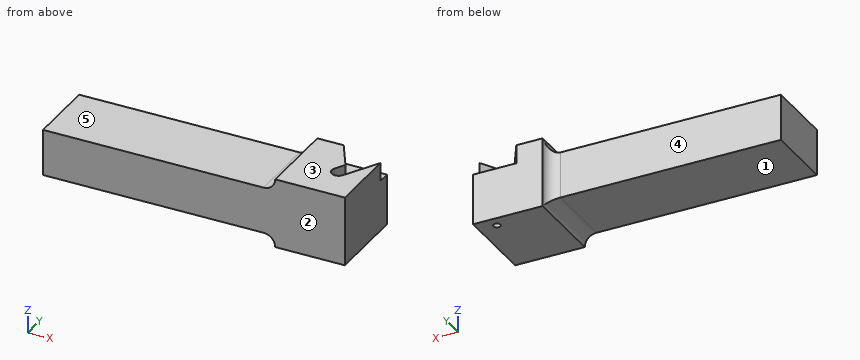
```python
from build123d import *

# Parameters (mm, degrees)
SKETCH_1_W          = 100
SKETCH_1_H          = 30
EXTRUDE_1_DEPTH     = 20
SKETCH_2_W          = 30
SKETCH_2_H          = 35
EXTRUDE_2_DEPTH     = 30
FILLET_1_R          = 5
CUT_EXTRUDE_1_DEPTH = 8
SKETCH_4_R          = 1.5
CUT_EXTRUDE_2_DEPTH = 91.049986119


with BuildPart() as part:
    # 草图1 → 凸台-拉伸1 (new body)
    with BuildSketch(Plane.XY):
        with Locations((5, 0)):
            Rectangle(SKETCH_1_W, SKETCH_1_H)
    extrude(amount=EXTRUDE_1_DEPTH)

    # 草图2 → 凸台-拉伸2 (add)
    with BuildSketch(Plane(origin=(55, 0, 0), x_dir=(0, 0, -1), z_dir=(1, 0, 0))):
        with Locations((-10, 2.5)):
            Rectangle(SKETCH_2_W, SKETCH_2_H)
    extrude(amount=EXTRUDE_2_DEPTH)

    # 圆角1
    fillet_1_edges = [part.edges().sort_by_distance(p)[0] for p in [
        (55, 0, 0),
        (55, 15, 10),
        (55, 0, 20),
    ]]
    fillet(fillet_1_edges, radius=FILLET_1_R - 0.0001)  # a hair under: the kernel refuses the full size

    # 草图3 → 切除-拉伸1 (cut)
    with BuildSketch(Plane.XY.offset(25)):
        with BuildLine():
            Line((73.842770799, 7.009618943), (66.342770799, 20))
            Line((66.342770799, 20), (85, 20))
            Line((85, 20), (85, 14.424396121))
            Line((85, 14.424396121), (78.356092757, 2.916811216))
            Line((78.356092757, 2.916811216), (76.5, -0.298035743))
            ThreePointArc((76.5, -0.298035743), (72.432621566, -1.38788651), (71.342770799, 2.679491924))
            Line((71.342770799, 2.679491924), (73.842770799, 7.009618943))
        make_face()
    extrude(amount=-CUT_EXTRUDE_1_DEPTH, mode=Mode.SUBTRACT)

    # 草图4 → 切除-拉伸2 (cut, through all)
    with BuildSketch(Plane.XY.offset(17)):
        with Locations((77.2809236, 15.014563609)):
            Circle(SKETCH_4_R)
    extrude(amount=-CUT_EXTRUDE_2_DEPTH, mode=Mode.SUBTRACT)


solid = part.part
```
Work out the finished part from the listing and answer in its coordinate system (mm). Face numbers are marked on the shaded views. A direction names the side the tool comes from. Give positions to 0.01 mm unless a question says otherwise; leave off trailing zeros. Write each loop counter-clockwise with the first axis right and the second up, starting at its lowest first coordinate (ties: lowest second). Pieces come first, ordered by that corner, then holes.
(1) The part is cut by section D-D on x = -35. Write down the section's boundary in (y, z).
Final values:
outline: (-15, 0) - (15, 0) - (15, 20) - (-15, 20) - close
(2) Straight lines are drawn through the part: line 1 (Z direction, x = -25.5, y = 1); line 2 (Y direction, x = 44.5, z = 1); line 3 (Y direction, x = 76.5, z = 13). For each, find the intervals that lie inside material, in ascending order.
Final values:
line 1: z = 0 to 20
line 2: y = -15 to 15
line 3: y = -15 to 13.73, 16.3 to 20
(3) Flat-ended cylindrical pins translate along their axes: pin 1 Ø8 at (x, y) = (18, -8) entering from -Z; pin 2 Ø16 at (x, z) = (25.5, 12.5) entering from +Y; pin 3 Ø9 at (x, y) = (18.5, 6.5) entering from +Z. Find the tip coordinate at first contact, or state that the pin passes through.
Final values:
pin 1: stops at z = 0
pin 2: stops at y = 15
pin 3: stops at z = 20
(4) Which of the six approach directions +Z, -Z, +X, -X, +Y, -Y give full straight-line access (tool end or side, diameter ignored) to the marked faces 1, 2, 3, 4 and 5?
Final values:
face 1: -Z, -X, +Y, -Y
face 2: +Z, -Z, +X, -X, -Y
face 3: +Z, +X, -X, +Y, -Y
face 4: +Z, -Z, -X, +Y
face 5: +Z, -X, +Y, -Y
